The model under review builds one solid part; all positions refer to its coordinate system, in mm. Round coordinates to 2 decimals unless told otherwise and drop trailing zeros. Write each loop counter-clockwise with the first axis right and the second up, starting at its lowest first coordinate (ties: lowest second). Pieces come first, ordered by that corner, then holes. Notation, with made-up numbers: (30, 7.5) -> (47, 7.5) arc R21 cw to (47, 45.5) -> close; hole circle Ø2 at (-13.5, 73.25). An arc over 180 degrees is marked (long way). Return JSON: item names as keys, results as strings. Group by question number.
1. Take a section at A-A, the plane x = 603.6. Write out the cut boundary in (y, z).
2. Take a section at B-B, the plane y = 253.5. Write out the cut boundary in (x, z), then the cut area to 3 significant figures.
3. For line 1 along Z through (x, y) = (601.95, 58); line 2 along Z through (x, y) = (602.45, 198); line 3 along Y through (x, z) = (602.75, 311), list the stretches that pass through material, from the lowest coordinate up. Write a range as from..to.
4. Clearance check with a flat-ended pin moving along its axis: P1, Ø1.5, axis at x = 603, y = 57.5, coming from the +Z side. State where the tip first meets the part, or that it passes through.
5. Take a section at C-C, the plane z = 329.5. Write out the cut boundary in (x, y).
from build123d import *

# Parameters (mm, degrees)
BOX006_W               = 18
BOX006_H               = 200
BOX006_DEPTH           = 87
BOX006_PLACEMENT_ANGLE = 30
BOX005_W               = 18
BOX005_H               = 200
BOX005_DEPTH           = 87
BOX005_PLACEMENT_ANGLE = 30
BOX004_W               = 348
BOX004_H               = 4
BOX004_DEPTH           = 400


with BuildPart() as box006:
    # Box006 → Box006 (new body)
    with BuildSketch(Plane.XY):
        with Locations((9, 100)):
            Rectangle(BOX006_W, BOX006_H)
    extrude(amount=BOX006_DEPTH)


with BuildPart() as box006_1:
    # Box006 placement: moved
    add(box006.part.moved(Location((598, 174.528857, 399.719854))).rotate(Axis((598, 174.528857, 399.719854), (-1, 0, 0)), BOX006_PLACEMENT_ANGLE))


with BuildPart() as glass_cut:
    # Box005 → Box005 (new body)
    with BuildSketch(Plane.XY):
        with Locations((9, 100)):
            Rectangle(BOX005_W, BOX005_H)
    extrude(amount=BOX005_DEPTH)


with BuildPart() as glass_cut_1:
    # Box005 placement: moved
    add(glass_cut.part.moved(Location((598, -0.25833, 301.447441))).rotate(Axis((598, -0.25833, 301.447441), (1, 0, 0)), BOX005_PLACEMENT_ANGLE))


with BuildPart() as glass_sides:
    # Box004 → Box004 (new body)
    with BuildSketch(Plane(origin=(605, 0, 0), x_dir=(0, 1, 0), z_dir=(0, 0, 1))):
        with Locations((174, 2)):
            Rectangle(BOX004_W, BOX004_H)
    extrude(amount=BOX004_DEPTH)

    # Cut: cut Glass cut
    add(glass_cut_1.part, mode=Mode.SUBTRACT)

    # Cut001: cut Box006
    add(box006_1.part, mode=Mode.SUBTRACT)


solid = glass_sides.part
Output:
{
 "1": {"outline": "(0, 0) -> (348, 0) -> (348, 300.18) -> (347.73, 299.72) -> (174.53, 399.72) -> (174.69, 400) -> (170.44, 400) -> (0, 301.6) -> close"},
 "2": {"outline": "(601, 0) -> (605, 0) -> (605, 354.13) -> (601, 354.13) -> close", "area": "1,420 mm^2"},
 "3": {"line 1": "z = 0..335.08", "line 2": "z = 0..386.17", "line 3": "y = 16.29..328.2"},
 "4": {"P1": "stops at z = 335.23"},
 "5": {"outline": "(601, 48.33) -> (605, 48.33) -> (605, 296.15) -> (601, 296.15) -> close"}
}
